Work out the finished part from the listing and answer in its coordinate system (mm). A direction names the side the tool comes from. Give positions to 0.01 mm unless a question says otherwise; leave off trailing zeros. Loops run counter-clockwise (first coordinate to the right, second up) from the corner with the lowest first, then second, coordinate; pieces in that order, holes last. Notation, with made-up numbers: (35.25, 35) - (82.25, 35) arc R31 ccw to (82.25, 74) - close; hole circle Ø4 at (58, 77). An arc over 180 degrees is marked (long way). Use CSV: the item, a comma, the result in double quotes.
from build123d import *

# Parameters (mm, degrees)
SKETCH1_R           = 0.6
BOSS_EXTRUDE1_DEPTH = 2.4
BOSS_EXTRUDE2_DEPTH = 3.8
BOSS_EXTRUDE3_DEPTH = 4


with BuildPart() as part:
    # Sketch1 → Boss-Extrude1 (new body)
    with BuildSketch(Plane.XY):
        with BuildLine():
            Line((1.240927797, 2.65), (-10.709121967, 1.99702088))
            ThreePointArc((-10.709121967, 1.99702088), (-12.6, 0), (-10.709121967, -1.99702088))
            Line((-10.709121967, -1.99702088), (1.240927797, -2.65))
            ThreePointArc((1.240927797, -2.65), (0, 0), (1.240927797, 2.65))
        make_face()
        with Locations((-1, 0)):
            Circle(SKETCH1_R, mode=Mode.SUBTRACT)
        with Locations((-3, 0)):
            Circle(SKETCH1_R, mode=Mode.SUBTRACT)
        with Locations((-5, 0)):
            Circle(SKETCH1_R, mode=Mode.SUBTRACT)
        with Locations((-7, 0)):
            Circle(SKETCH1_R, mode=Mode.SUBTRACT)
        with Locations((-9, 0)):
            Circle(SKETCH1_R, mode=Mode.SUBTRACT)
        with Locations((-11, 0)):
            Circle(SKETCH1_R, mode=Mode.SUBTRACT)
    extrude(amount=BOSS_EXTRUDE1_DEPTH)

    # Sketch1_4 → Boss-Extrude2 (add)
    with BuildSketch(Plane.XY):
        with BuildLine():
            Line((-10.709121967, 1.99702088), (-30.711406288, 0.904048527))
            ThreePointArc((-30.711406288, 0.904048527), (-31.615454815, 0), (-30.711406288, -0.904048527))
            Line((-30.711406288, -0.904048527), (-10.709121967, -1.99702088))
            ThreePointArc((-10.709121967, -1.99702088), (-12.6, 0), (-10.709121967, 1.99702088))
        make_face()
        with BuildLine():
            Line((-13.478774997, 0.844188674), (-28.928115358, 0))
            Line((-28.928115358, 0), (-13.478774997, -0.844188674))
            ThreePointArc((-13.478774997, -0.844188674), (-13.6, 0), (-13.478774997, 0.844188674))
        make_face(mode=Mode.SUBTRACT)
    extrude(amount=BOSS_EXTRUDE2_DEPTH)

    # Sketch2 → Boss-Extrude3 (add)
    with BuildSketch(Plane(origin=(0, 0, 0), x_dir=(-1, 0, 0), z_dir=(0, 0, -1))):
        with BuildLine():
            Line((12.484683103, 0.843865841), (12.484683103, -0.843865841))
            ThreePointArc((12.484683103, -0.843865841), (12.797137099, -1.570006662), (13.539244087, -1.842376282))
            Line((13.539244087, -1.842376282), (30.711406288, -0.904048527))
            ThreePointArc((30.711406288, -0.904048527), (31.615454815, 0), (30.711406288, 0.904048527))
            Line((30.711406288, 0.904048527), (13.539244087, 1.842376282))
            ThreePointArc((13.539244087, 1.842376282), (12.797137099, 1.570006662), (12.484683103, 0.843865841))
        make_face()
        with BuildLine():
            Line((28.928115358, 0), (13.478774997, -0.844188674))
            ThreePointArc((13.478774997, -0.844188674), (13.6, 0), (13.478774997, 0.844188674))
            Line((13.478774997, 0.844188674), (28.928115358, 0))
        make_face(mode=Mode.SUBTRACT)
    extrude(amount=BOSS_EXTRUDE3_DEPTH)


solid = part.part
Item 1: For faces 4 (the flat face through (-12.485, 0, -2)), 5 (the cylindrical face through (-0.428, 0.18, 1.183)), determine the directions among +Z, -Z, +X, -X, +Y, -Y from which every point of the face is accessible in a straight line to the end or side of a thin tool.
Determined:
face 4,"-Z, +X, +Y, -Y"
face 5,"+Z, -Z"
Item 2: A cutting plane is placed at C-C on z = 0.5. Determine the outline of the cut face in (x, y), and give its area (3 significant figures).
Determined:
outline,"(-30.71, -0.9) - (1.24, -2.65) arc R3.45 cw to (1.24, 2.65) - (-30.71, 0.9) arc R0.9 ccw to start; hole (-28.93, 0) - (-13.48, -0.84) arc R3 cw to (-13.48, 0.84) - close; hole circle Ø1.2 at (-11, 0); hole circle Ø1.2 at (-9, 0); hole circle Ø1.2 at (-7, 0); hole circle Ø1.2 at (-5, 0); hole circle Ø1.2 at (-3, 0); hole circle Ø1.2 at (-1, 0)"
area,"90.6 mm²"
Item 3: A cutting plane is placed at A-A on x = -16.5. Determine the outline of the cut face in (y, z), and give its area (3 significant figures).
Determined:
outline,"(-1.68, -4) - (-0.68, -4) - (-0.68, 3.8) - (-1.68, 3.8) - close; (0.68, -4) - (1.68, -4) - (1.68, 3.8) - (0.68, 3.8) - close"
area,"15.6 mm²"
Item 4: Given P1, Ø0.5, axis at y = 0, z = -1.5, coming from the +X side; P2, Ø1.9, axis at x = -5, y = 0, coming from the +Z side; P3, Ø1.9, axis at x = -11, y = 0, coming from the -Z side, each flat-ended and moving along its own axis, determine where each tip first touches the part or whether it passes through.
Determined:
P1,"stops at x = -12.48"
P2,"stops at z = 2.4"
P3,"stops at z = 0"
Item 5: Find the intervals of material crossed by line 1 (Y direction, x = -5, z = 0.7); line 2 (Y direction, x = -25, z = 3.75); line 3 (Z direction, x = -12, y = -0.25), in increasing order.
Determined:
line 1,"y = -2.31 to -0.6, 0.6 to 2.31"
line 2,"y = -1.22 to -0.21, 0.21 to 1.22"
line 3,"z = 0 to 2.4"
Item 6: The mould has two halves that part along X. Classify faces 1 (the flat face through (-21, -1, 3.8)), 2 (the cylindrical face through (-12.6, 0, 3.1)), 3 (the flat face through (-21.095, 0.428, -0.045)): pulls with the +X half, pulls with the -X half, needs draft (parallel to the pull), parting line crosses it, or undercut.
Determined:
face 1,"needs draft"
face 2,"pulls with the +X half"
face 3,"undercut"
Item 7: A cutting plane is placed at D-D on x = -1. Determine the outline of the cut face in (y, z), and give its area (3 significant figures).
Determined:
outline,"(-2.53, 0) - (-0.6, 0) - (-0.6, 2.4) - (-2.53, 2.4) - close; (0.6, 0) - (2.53, 0) - (2.53, 2.4) - (0.6, 2.4) - close"
area,"9.25 mm²"
Item 8: A cutting plane is placed at B-B on z = -2.25. Determine the outline of the cut face in (x, y), and give its area (3 significant figures).
Determined:
outline,"(-30.71, -0.9) - (-13.54, -1.84) arc R1 ccw to (-12.48, -0.84) - (-12.48, 0.84) arc R1 ccw to (-13.54, 1.84) - (-30.71, 0.9) arc R0.9 ccw to start; hole (-28.93, 0) - (-13.48, -0.84) arc R3 cw to (-13.48, 0.84) - close"
area,"39.0 mm²"
